Geometry: final body of the model. Coordinates: model frame, mm. A direction names the side the tool comes from. Round coordinates to 2 decimals unless told otherwise and drop trailing zeros. Loops run counter-clockwise (first coordinate to the right, second up) from the corner with the lowest first, then second, coordinate; pieces in that order, holes last. Notation, with made-up numbers: M 76,60 L 109,60 A18 cw 109,91 Z; hole C 23.5,23.25 d8. An arc over 180 degrees is marked long. Answer as a JSON object with one key per item and string values.
```python
from build123d import *

# Parameters (mm, degrees)
ESQUISSE1_R             = 1.5
BOSS_EXTRU_1_DEPTH      = 5
ESQUISSE2_W             = 20
ESQUISSE2_H             = 20
ENL_V_MAT_EXTRU_1_DEPTH = 114.247516529
ESQUISSE3_R             = 1
ENL_V_MAT_EXTRU_2_DEPTH = 114.247516529


with BuildPart() as part:
    # Esquisse1 → Boss.-Extru.1 (new body)
    with BuildSketch(Plane.XY):
        with BuildLine():
            Line((40, 50), (40, 80))
            Line((40, 80), (5, 80))
            ThreePointArc((5, 80), (1.464466094, 78.535533906), (0, 75))
            Line((0, 75), (0, 5))
            ThreePointArc((0, 5), (1.464466094, 1.464466094), (5, 0))
            Line((5, 0), (40, 0))
            Line((40, 0), (40, 30))
            Line((40, 30), (40, 50))
        make_face()
        with Locations((25.6, 76)):
            Circle(ESQUISSE1_R, mode=Mode.SUBTRACT)
        with Locations((25.6, 4)):
            Circle(ESQUISSE1_R, mode=Mode.SUBTRACT)
    boss_extru_1 = extrude(amount=BOSS_EXTRU_1_DEPTH)

    # Symétrie1: Boss.-Extru.1 across plane
    add(boss_extru_1.mirror(Plane(origin=(40, 50, 5), x_dir=(0, 0, 1), z_dir=(-1, 0, 0))))

    # Esquisse2 → Enlèv. mat.-Extru.1 (cut, through all)
    with BuildSketch(Plane.XY.offset(5)):
        with Locations((40.6, 40)):
            Rectangle(ESQUISSE2_W, ESQUISSE2_H)
    extrude(amount=-ENL_V_MAT_EXTRU_1_DEPTH, mode=Mode.SUBTRACT)

    # Esquisse3 → Enlèv. mat.-Extru.2 (cut, through all)
    with BuildSketch(Plane.XY.offset(5)):
        with Locations((54, 36)):
            Circle(ESQUISSE3_R)
        with Locations((54, 16)):
            Circle(ESQUISSE3_R)
        with Locations((36, 26)):
            Circle(ESQUISSE3_R)
        with Locations((16, 26)):
            Circle(ESQUISSE3_R)
    extrude(amount=-ENL_V_MAT_EXTRU_2_DEPTH, mode=Mode.SUBTRACT)


solid = part.part
```
1) Cut plane B-B on x = 32.5. Return the cut outline in (y, z).
Geometry results:
{"outline": "M 0,0 L 30,0 L 30,5 L 0,5 Z; M 50,0 L 80,0 L 80,5 L 50,5 Z"}
2) Cut plane C-C on z = 2.15. Count the separate pieces of the cut face and the enclosed holes in it, and give its area (3 significant figures).
Geometry results:
{"separate pieces": "1", "enclosed holes": "9", "area": "5,940 mm2"}
3) Cut plane A-A on y = 16. Return the cut outline in (x, z), and give its area (3 significant figures).
Geometry results:
{"outline": "M 0,0 L 53,0 L 53,5 L 0,5 Z; M 55,0 L 80,0 L 80,5 L 55,5 Z", "area": "390 mm2"}
4) Set-up query: faces 1 (the face through (78, 79, 2)), 2 (the face through (40, 30, 3)). Return all of +Z, -Z, +X, -X, +Y, -Y with unobstructed straight access to the full face (end or side cutting, diameter ignored); none if empty.
Geometry results:
{"face 1": "+Z, -Z, +X, +Y", "face 2": "+Z, -Z"}
5) Pull-direction query (X, two-part tool) for faces 3 (the face through (25.405, 77.487, 2.465)), 4 (the face through (23, 41, 5)), 5 (the face through (0, 40, 2)); classes: +X half, -X half, draft (parallel to the pull), parting line (faces both ways), or undercut.
Geometry results:
{"face 3": "undercut", "face 4": "draft", "face 5": "-X half"}
6) Cut plane D-D on y = 26. Return the cut outline in (x, z).
Geometry results:
{"outline": "M 0,0 L 15,0 L 15,5 L 0,5 Z; M 17,0 L 35,0 L 35,5 L 17,5 Z; M 37,0 L 80,0 L 80,5 L 37,5 Z"}
7) Line query: probe 1 along Y at (x, z) = (25.6, 2.65); probe 2 along X at (y, z) = (38, 0.75); probe 3 along Y at (x, z) = (33, 3.05). Output: solid intervals per line, ascending.
Geometry results:
{"probe 1": "0 to 2.5, 5.5 to 74.5, 77.5 to 80", "probe 2": "0 to 30.6, 50.6 to 80", "probe 3": "0 to 30, 50 to 80"}
